```python
from build123d import *

# Parameters (mm, degrees)
SKETCH_1_W      = 31.8
SKETCH_1_H      = 20.3
EXTRUDE_1_DEPTH = 10.2
FILLET_2_R      = 1
FILLET_1_R      = 3
SKETCH_2_R      = 0.25
EXTRUDE_2_DEPTH = 3.05


with BuildPart() as part:
    # Эскиз1 → Бобышка-Вытянуть1 (new body)
    with BuildSketch(Plane.XY):
        Rectangle(SKETCH_1_W, SKETCH_1_H)
    extrude(amount=EXTRUDE_1_DEPTH)

    # Скругление2
    fillet_2_edges = [part.edges().sort_by_distance(p)[0] for p in [
        (-15.9, 0, 10.2),
        (0, -10.15, 10.2),
        (15.9, 0, 10.2),
        (0, -10.15, 0),
        (-15.9, 0, 0),
        (0, 10.15, 0),
        (15.9, 0, 0),
        (0, 10.15, 10.2),
    ]]
    fillet(fillet_2_edges, radius=FILLET_2_R)

    # Скругление1
    # the kernel refuses this fillet: 3 mm, written as the material it takes off along each edge
    with BuildSketch(Plane(origin=(12.9, -7.15, 0), x_dir=(1, 0, 0), z_dir=(0, 1, 0))) as fillet_1_piece_1:
        with BuildLine():
            CenterArc((2, -1), 1, 0, 90)
            Line((3, -1), (3, 0))
            Line((3, 0), (2, 0))
        make_face()
    revolve(axis=Axis((12.9, -7.15, 0), (0, 0, -1)), revolution_arc=90, mode=Mode.SUBTRACT)
    with BuildSketch(Plane(origin=(-12.9, -7.15, 0), x_dir=(0, -1, 0), z_dir=(1, 0, 0))) as fillet_1_piece_2:
        with BuildLine():
            CenterArc((2, -1), 1, 0, 90)
            Line((3, -1), (3, 0))
            Line((3, 0), (2, 0))
        make_face()
    revolve(axis=Axis((-12.9, -7.15, 0), (0, 0, -1)), revolution_arc=90, mode=Mode.SUBTRACT)
    with BuildSketch(Plane(origin=(12.9, 7.15, 0), x_dir=(0, 1, 0), z_dir=(-1, 0, 0))) as fillet_1_piece_3:
        with BuildLine():
            CenterArc((2, -1), 1, 0, 90)
            Line((3, -1), (3, 0))
            Line((3, 0), (2, 0))
        make_face()
    revolve(axis=Axis((12.9, 7.15, 0), (0, 0, -1)), revolution_arc=90, mode=Mode.SUBTRACT)
    with BuildSketch(Plane(origin=(-12.9, 7.15, 0), x_dir=(-1, 0, 0), z_dir=(0, -1, 0))) as fillet_1_piece_4:
        with BuildLine():
            CenterArc((2, -1), 1, 0, 90)
            Line((3, -1), (3, 0))
            Line((3, 0), (2, 0))
        make_face()
    revolve(axis=Axis((-12.9, 7.15, 0), (0, 0, -1)), revolution_arc=90, mode=Mode.SUBTRACT)
    with BuildSketch(Plane(origin=(12.9, -7.15, 10.2), x_dir=(0, -1, 0), z_dir=(-1, 0, 0))) as fillet_1_piece_5:
        with BuildLine():
            CenterArc((2, -1), 1, 0, 90)
            Line((3, -1), (3, 0))
            Line((3, 0), (2, 0))
        make_face()
    revolve(axis=Axis((12.9, -7.15, 10.2), (0, 0, 1)), revolution_arc=90, mode=Mode.SUBTRACT)
    with BuildSketch(Plane(origin=(-12.9, -7.15, 10.2), x_dir=(-1, 0, 0), z_dir=(0, 1, 0))) as fillet_1_piece_6:
        with BuildLine():
            CenterArc((2, -1), 1, 0, 90)
            Line((3, -1), (3, 0))
            Line((3, 0), (2, 0))
        make_face()
    revolve(axis=Axis((-12.9, -7.15, 10.2), (0, 0, 1)), revolution_arc=90, mode=Mode.SUBTRACT)
    with BuildSketch(Plane(origin=(12.9, 7.15, 10.2), x_dir=(1, 0, 0), z_dir=(0, -1, 0))) as fillet_1_piece_7:
        with BuildLine():
            CenterArc((2, -1), 1, 0, 90)
            Line((3, -1), (3, 0))
            Line((3, 0), (2, 0))
        make_face()
    revolve(axis=Axis((12.9, 7.15, 10.2), (0, 0, 1)), revolution_arc=90, mode=Mode.SUBTRACT)
    with BuildSketch(Plane(origin=(-12.9, 7.15, 10.2), x_dir=(0, 1, 0), z_dir=(1, 0, 0))) as fillet_1_piece_8:
        with BuildLine():
            CenterArc((2, -1), 1, 0, 90)
            Line((3, -1), (3, 0))
            Line((3, 0), (2, 0))
        make_face()
    revolve(axis=Axis((-12.9, 7.15, 10.2), (0, 0, 1)), revolution_arc=90, mode=Mode.SUBTRACT)
    with BuildSketch(Plane(origin=(-15.9, 10.15, 0), x_dir=(0, -1, 0), z_dir=(0, 0, 1)), Plane(origin=(-15.9, -10.15, 0), x_dir=(1, 0, 0), z_dir=(0, 0, 1))) as fillet_1_piece_9:
        with BuildLine():
            CenterArc((FILLET_1_R, FILLET_1_R), FILLET_1_R, 180, 90)
            Line((0, FILLET_1_R), (0, 0))
            Line((0, 0), (FILLET_1_R, 0))
        make_face()
    extrude(amount=10.2, mode=Mode.SUBTRACT)
    with BuildSketch(Plane(origin=(15.9, 10.15, 0), x_dir=(0, -1, 0), z_dir=(0, 0, 1)), Plane(origin=(15.9, -10.15, 0), x_dir=(-1, 0, 0), z_dir=(0, 0, 1))) as fillet_1_piece_10:
        with BuildLine():
            CenterArc((FILLET_1_R, -FILLET_1_R), FILLET_1_R, 90, 90)
            Line((0, -FILLET_1_R), (0, 0))
            Line((0, 0), (FILLET_1_R, 0))
        make_face()
    extrude(amount=10.2, mode=Mode.SUBTRACT)

    # Эскиз2 → Бобышка-Вытянуть2 (add)
    with BuildSketch(Plane(origin=(0, 0, 0), x_dir=(-1, 0, 0), z_dir=(0, 0, -1))):
        with Locations((13.98, 7.62)):
            Circle(SKETCH_2_R)
        with Locations((8.9, 7.62)):
            Circle(SKETCH_2_R)
        with Locations((-11.44, 7.62)):
            Circle(SKETCH_2_R)
        with Locations((-13.98, 7.62)):
            Circle(SKETCH_2_R)
        with Locations((-13.98, -7.62)):
            Circle(SKETCH_2_R)
        with Locations((-11.44, -7.62)):
            Circle(SKETCH_2_R)
        with Locations((8.9, -7.62)):
            Circle(SKETCH_2_R)
        with Locations((13.98, -7.62)):
            Circle(SKETCH_2_R)
        with Locations((-8.9, 7.62)):
            Circle(SKETCH_2_R)
        with Locations((-8.9, -7.62)):
            Circle(SKETCH_2_R)
        with Locations((11.44, 7.62)):
            Circle(SKETCH_2_R)
        with Locations((11.44, -7.62)):
            Circle(SKETCH_2_R)
    extrude(amount=EXTRUDE_2_DEPTH)


solid = part.part
```
The listing builds one solid part. Answer for the finished solid, in the listing's coordinates (mm). Give positions to 0.01 mm unless a question says otherwise; leave off trailing zeros. Loops run counter-clockwise (first coordinate to the right, second up) from the corner with the lowest first, then second, coordinate; pieces in that order, holes last. Notation, with made-up numbers: (4, 49) - (19, 49) arc R14 cw to (19, 62) - close; hole circle Ø9 at (65, -26.75). An arc over 180 degrees is marked (long way). Return JSON: item names as keys, results as strings. Group by question number.
1. Straight lines are drawn through the part: line 1 (X direction, y = 7.5, z = -2.5); line 2 (Z direction, x = -2, y = -6); line 3 (Y direction, x = -13, z = 7.5). For each, find the intervals that lie inside material, in ascending order. Write a range as [from, to].
2. Find section A-A (z = -0.75). State how many separate pieces and enclosed holes the cut face has, then the cut area to 3 significant figures.
3. Given pin 1 Ø3 at (x, y) = (-10, 6) entering from -Z, flat-ended and moving along its own axis, determine where the tip first touches the part or whether it passes through.
4. Find section B-B (y = 4). Write down the section's boundary in (x, z), then the cut area to 3 significant figures.
Verdict:
{
 "1": {"line 1": "x = [-14.2, -13.76], [-11.66, -11.22], [-9.12, -8.68], [8.68, 9.12], [11.22, 11.66], [13.76, 14.2]", "line 2": "z = [0, 10.2]", "line 3": "y = [-10.15, 10.15]"},
 "2": {"separate pieces": "12", "enclosed holes": "0", "area": "2.36 mm^2"},
 "3": {"pin 1": "stops at z = 0"},
 "4": {"outline": "(-15.9, 1) arc R1 ccw to (-14.9, 0) - (14.9, 0) arc R1 ccw to (15.9, 1) - (15.9, 9.2) arc R1 ccw to (14.9, 10.2) - (-14.9, 10.2) arc R1 ccw to (-15.9, 9.2) - close", "area": "324 mm^2"}
}
